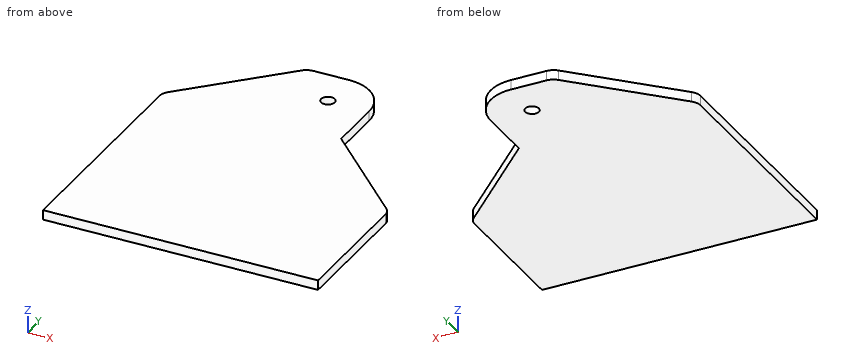
Autodesk Inventor part; units mm, degrees
ref_plane "YZ Plane" through (0, 0, 0) normal (1, 0, 0) x (0, 1, 0)
ref_plane "XZ Plane" through (0, 0, 0) normal (0, 1, 0) x (-1, 0, 0)
ref_plane "XY Plane" through (0, 0, 0) normal (0, 0, 1) x (1, 0, 0)
sketch "Sketch1" plane through (0, 0, 0) normal (0, 0, 1) x (1, 0, 0)
  line L0 (0, 0) -> (508, 0)
  line L1 (508, 0) -> (508, 609.6)
  line L2 (508, 609.6) -> (0, 609.6)
  line L3 (0, 609.6) -> (0, 0)
  line L4 (254, 609.6) -> (177.8, 609.6)
  line L5 (177.8, 609.6) -> (125.7631, 609.6)
  line L6 (254, 609.6) -> (330.2, 609.6)
  line L7 (177.8, 609.6) -> (0, 431.8)
  line L8 (177.8, 609.6) -> (429.2472, 609.6) construction
  line L9 (330.2, 609.6) -> (330.2, 431.8)
  line L10 (330.2, 431.8) -> (508, 254)
  circle A0 centre (254, 533.4) radius 12.7
  dimension "d0" = 508
  dimension "d1" = 609.6
  dimension "d2" = 76.2
  dimension "d3" = 76.2
  dimension "d4" = 135
  dimension "d5" = 135
  dimension "d6" = 25.4
  dimension "d7" = 76.2
  dimension "d10" = 177.8
  dimension "d11" = 538.8154
  dimension "d12" = 254
  dimension "d13" = 382.2369
  dimension "d14" = 254
extrude "Extrusion1" add sketch "Sketch1" along normal blind 18.0086 contours L3 L7 L2 L9 L10 L1 L0
fillet "Fillet1" radius 76.2 1 edges at (330.2, 609.6, 9.0043)
fillet "Fillet2" radius 25.4 1 edges at (177.8, 609.6, 9.0043)
fillet "Fillet3" radius 25.4 1 edges at (0, 431.8, 9.0043)
fillet "Fillet4" radius 25.4 1 edges at (508, 254, 9.0043)
properties part number "base side"
Part model, mm, in its own coordinate system. Coordinates: 2 decimals unless noted, no trailing zeros. Write each loop counter-clockwise with the first axis right and the second up, starting at its lowest first coordinate (ties: lowest second). Pieces come first, ordered by that corner, then holes. Notation, with made-up numbers: M 9.5,-13 L 33.5,-13 A19 cw 33.5,10 Z; hole C 12,11 d9. An arc over 180 degrees is marked long. Return JSON: item names as keys, results as strings.
1. Saw through at B-B, the plane y = 454. Write the cut outline in (x, z).
Determined:
{"outline": "M 22.2,0 L 330.2,0 L 330.2,18.01 L 22.2,18.01 Z"}
2. Saw through at A-A, the plane z = 5.75. Write the cut outline in (x, y), then the cut area to 3 significant figures.
Determined:
{"outline": "M 0,0 L 508,0 L 508,243.48 A25.4 ccw 500.56,261.44 L 330.2,431.8 L 330.2,533.4 A76.2 ccw 254,609.6 L 188.32,609.6 A25.4 ccw 170.36,602.16 L 7.44,439.24 A25.4 ccw 0,421.28 Z; hole C 254,533.4 d25.4", "area": "245,000 mm²"}
3. Probe L1, parallel to Y at x = 254, z = 6.5; L2, parallel to X at y = 533.4, z = 6.25; L3, parallel to X at y = 284, z = 9. List the from-to ranges inside material, lowest first.
Determined:
{"L1": "0 to 520.7, 546.1 to 609.6", "L2": "101.6 to 241.3, 266.7 to 330.2", "L3": "0 to 478"}
4. Flat gauge pins, fed straight in: pin 1 Ø5 at (y, z) = (141.5, 2.5) entering from -X; pin 2 Ø6 at (y, z) = (544, 12.5) entering from -X; pin 3 Ø15 at (x, y) = (254, 533.4) entering from +Z; pin 4 Ø6 at (y, z) = (545, 10) entering from -X. Where does each tip first touch, or does it go through?
Determined:
{"pin 1": "x = 0", "pin 2": "x = 109.2", "pin 3": "through", "pin 4": "x = 110.2"}
5. Saw through at C-C, the plane x = 41. Write the cut outline in (y, z).
Determined:
{"outline": "M 0,0 L 472.8,0 L 472.8,18.01 L 0,18.01 Z"}
